from build123d import *

# Parameters (mm, degrees)
SKETCH1_R           = 9.525
BOSS_EXTRUDE1_DEPTH = 33.3375
CHAMFER1_SIZE       = 1.524


with BuildPart() as part:
    # Sketch1 → Boss-Extrude1 (new, symmetric)
    with BuildSketch(Plane.XY):
        Circle(SKETCH1_R)
    extrude(amount=BOSS_EXTRUDE1_DEPTH, both=True)

    # Chamfer1
    chamfer1_edges = [part.edges().sort_by_distance(p)[0] for p in [
        (-9.525, 0, -33.3375),
        (-9.525, 0, 33.3375),
    ]]
    chamfer(chamfer1_edges, length=CHAMFER1_SIZE)

    # Sketch3 → 1/4-20 Tapped Hole1 (revolve, cut)
    with BuildSketch(Plane(origin=(-9.525, 0, -22.225), x_dir=(0, 0, 1), z_dir=(0, 1, 0))):
        Polygon((0, 0), (0, 19.05), (3.81, 19.05), (2.5527, 17.7927), (2.5527, 1.2573), (3.81, 0), align=None)
    revolve(axis=Axis((-15.875, 0, -22.225), (1, 0, 0)), mode=Mode.SUBTRACT)

    # Groove Sketch → Retaining Ring Groove (revolve, cut)
    with BuildSketch(Plane(origin=(9.513189126, 2.614578126, 39.123243658), x_dir=(-0.3010163797724101, -0.08273049466574514, 0.9500235809500064), z_dir=(0.26501052487715226, -0.9642455194110764, 0)), mode=Mode.PRIVATE) as retaining_ring_groove_sk:
        with BuildLine():
            Line((-1.782805189, 20.756214823), (-1.711441265, 20.973390213))
            Line((-1.711441265, 20.973390213), (-3.2075384, 21.46500836))
            Line((-3.2075384, 21.46500836), (-3.278902324, 21.247832969))
            ThreePointArc((-3.278902324, 21.247832969), (-3.271598278, 21.150906191), (-3.197895954, 21.08753335))
            Line((-3.197895954, 21.08753335), (-1.943104809, 20.675208453))
            ThreePointArc((-1.943104809, 20.675208453), (-1.84617803, 20.682512499), (-1.782805189, 20.756214823))
        make_face()
    revolve(retaining_ring_groove_sk.sketch.rotate(Axis((0, 0, 54.757401128), (0, 0, -1)), 15.367578188), axis=Axis((0, 0, 54.757401128), (0, 0, -1)), mode=Mode.SUBTRACT)


solid = part.part
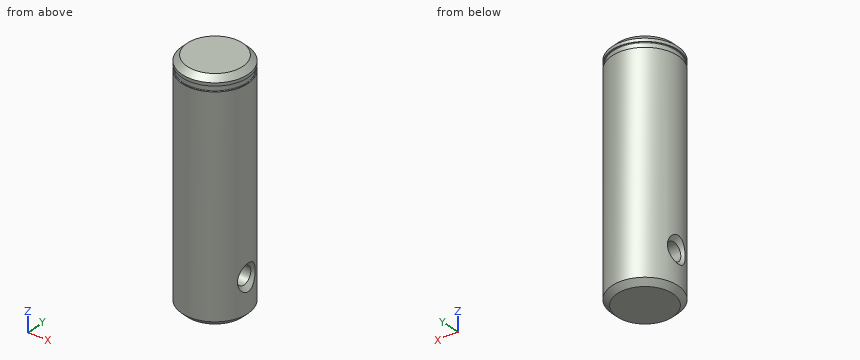
Input: part model. Units: mm. Frame: model coordinates. Coordinates: 2 decimals unless noted, no trailing zeros. Loops run counter-clockwise (first coordinate to the right, second up) from the corner with the lowest first, then second, coordinate; pieces in that order, holes last. Notation, with made-up numbers: (29, -18) - (69, -18) arc R12 cw to (69, 3) - close; hole circle Ø1 at (13, 39). An arc over 180 degrees is marked (long way). Answer in a Markdown table with one row per item. Add a question column.
Item 1: Line query: line 1 along Z through (x, y) = (0.5, 0); line 2 along Y through (x, z) = (-0.5, -12.5); line 3 along Z through (x, y) = (8.75, -1.5). Output: solid intervals per line, ascending. Write a range as [from, to].
Item 2: Section query C-C on z = -16. Return the cut outline in (x, y) (3 decimals).
Item 3: Contact query for flat-ended pins moving along their axis: P1, Ø1.5, axis at x = 1, z = 9.5, coming from the +Y side; P2, Ø2, axis at x = -3, z = -15.5, coming from the +Y side; P3, Ø1, axis at x = 3, z = 7.5, coming from the -Y side. Output: stop coordinate, or through.
Recorded:
| question | item | result |
|---|---|---|
| 1 | line 1 | [-33.34, -24.78], [-19.67, 33.34] |
| 1 | line 2 | [-9.51, 9.51] |
| 1 | line 3 | [-32.46, -24.86], [-19.59, 32.46] |
| 2 | outline | circle Ø19.05 at (0, 0) |
| 3 | P1 | y = 9.52 |
| 3 | P2 | y = 9.31 |
| 3 | P3 | y = -9.19 |
